```python
from build123d import *

# Parameters (mm, degrees)
F1_DEPTH = 12
F3_DEPTH = 90


with BuildPart() as f1:
    # F0 (on Front) → F1 (new body)
    with BuildSketch(Plane.XZ):
        Polygon((47.5, -67), (47.5, 0), (47.5, 67), (0, 67), (-47.5, 67), (-47.5, -67), align=None)
    extrude(amount=F1_DEPTH)

    # F2 (on face) → F3 (join)
    with BuildSketch(Plane.XZ.offset(12)):
        with BuildLine():
            Line((0, 5), (0, 0))
            Line((0, 0), (-4.8013158464, 0))
            ThreePointArc((-4.8013158464, 0), (-1.2386876382, -6.0708472044), (0, -13))
            ThreePointArc((0, -13), (12.7279220614, -7.7279220614), (18, 5))
            ThreePointArc((18, 5), (12.7279220614, 17.7279220614), (0, 23))
            Line((0, 23), (0, 5))
        make_face()
        with BuildLine():
            Line((-4.8013158464, 0), (0, 0))
            Line((0, 0), (0, 5))
            Line((0, 5), (0, 23))
            ThreePointArc((0, 23), (-5.397234005, 11.476680806), (-17.7049180328, 8.2459016393))
            ThreePointArc((-17.7049180328, 8.2459016393), (-17.8156486606, 7.5695647107), (-17.9005524862, 6.8895027624))
            ThreePointArc((-17.9005524862, 6.8895027624), (-10.6901851858, 4.7010550004), (-4.8013158464, 0))
        make_face()
        with BuildLine():
            ThreePointArc((0, -13), (-1.2386876382, -6.0708472044), (-4.8013158464, 0))
            Line((-4.8013158464, 0), (-7.550100402, 0))
            ThreePointArc((-7.550100402, 0), (-3.4675400893, -5.881167982), (-2.0003453113, -12.8885052096))
            ThreePointArc((-2.0003453113, -12.8885052096), (-1.0017250687, -12.9721046872), (0, -13))
        make_face()
        with BuildLine():
            Line((-7.550100402, 0), (-4.8013158464, 0))
            ThreePointArc((-4.8013158464, 0), (-10.6901851858, 4.7010550004), (-17.9005524862, 6.8895027624))
            ThreePointArc((-17.9005524862, 6.8895027624), (-17.9779647514, 5.8903838491), (-17.9996546887, 4.8885052096))
            ThreePointArc((-17.9996546887, 4.8885052096), (-12.3726305137, 3.3040864423), (-7.550100402, 0))
        make_face()
        with BuildLine():
            ThreePointArc((-2.0003453113, -12.8885052096), (-3.4675400893, -5.881167982), (-7.550100402, 0))
            Line((-7.550100402, 0), (-17.2916164658, 0))
            ThreePointArc((-17.2916164658, 0), (-11.6005749399, -8.76323585), (-2.0003453113, -12.8885052096))
        make_face()
        with BuildLine():
            Line((-17.2916164658, 0), (-7.550100402, 0))
            ThreePointArc((-7.550100402, 0), (-12.3726305137, 3.3040864423), (-17.9996546887, 4.8885052096))
            ThreePointArc((-17.9996546887, 4.8885052096), (-17.8141187186, 2.4198499502), (-17.2916164658, 0))
        make_face()
        with BuildLine():
            ThreePointArc((-17.7049180328, 8.2459016393), (-5.397234005, 11.476680806), (0, 23))
            ThreePointArc((0, 23), (-1.0017918512, 22.9721009647), (-2.0004782551, 22.888490343))
            ThreePointArc((-2.0004782551, 22.888490343), (-6.6776028044, 13.0131233652), (-17.2344944225, 10.1934768701))
            ThreePointArc((-17.2344944225, 10.1934768701), (-17.4968253692, 9.2262396998), (-17.7049180328, 8.2459016393))
        make_face()
        with BuildLine():
            ThreePointArc((-17.2344944225, 10.1934768701), (-6.6776028044, 13.0131233652), (-2.0004782551, 22.888490343))
            ThreePointArc((-2.0004782551, 22.888490343), (-11.523319194, 18.8279830328), (-17.2344944225, 10.1934768701))
        make_face()
    extrude(amount=F3_DEPTH)


solid = f1.part
```
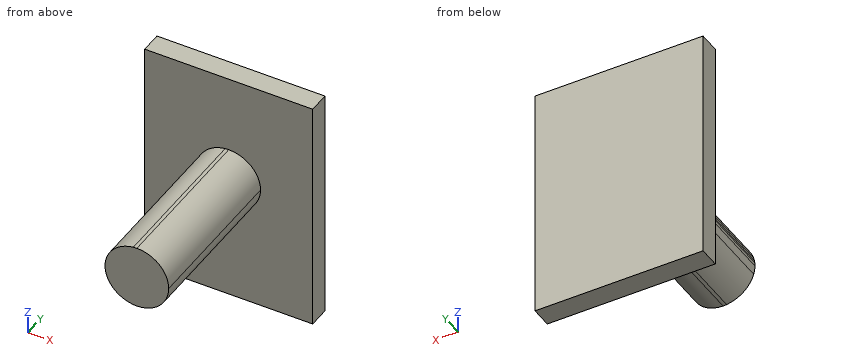
Design review of the part built by this model. Coordinates are the model's own, in mm. Coordinates: 2 decimals unless noted, no trailing zeros. Order: outer loops, then holes, each group sorted by start corner. A loop starts at its lowest first (then second) coordinate and runs counter-clockwise, first axis right, second up.
1) Wall thickness on line 1 along Y through (x, z) = (41, -47); line 2 along X through (y, z) = (-68.5, 18); line 3 along Z through (x, y) = (-11, -84): over which ranges is each line inside the solid? List them lowest first.
2) Take a section at B-B, the plane x = 13. Give the boundary of the cut face in (y, z), and give its area (3 significant figures).
3) Take a section at A-A, the plane y = -18. Give the boundary of the cut face in (x, z), and give its area (3 significant figures).
4) Take a section at D-D, the plane x = -26.5. Give the boundary of the cut face in (y, z).
5) Clearance check with flat-ended pins moving along their axes: pin 1 (10 mm diameter, centred on x = -33, z = 43, fed in from -Y); pin 2 (1 mm diameter, centred on x = -12, y = -43.5, fed in from -Z); pin 3 (12 mm diameter, centred on y = -44, z = 15, fed in from +X). State where each tip first meets the part, or that it passes through.
6) Take a section at C-C, the plane z = 14.5. Give the boundary of the cut face in (x, y), and give its area (3 significant figures).
Returned:
1. line 1: y = -12 to 0
1. line 2: x = -12.45 to 12.45
1. line 3: z = -9.25 to 19.25
2. outline: (-102, -7.45) - (-12, -7.45) - (-12, -67) - (0, -67) - (0, 67) - (-12, 67) - (-12, 17.45) - (-102, 17.45) - close
2. area: 3,850 mm2
3. outline: circle Ø36 at (0, 5)
3. area: 1,020 mm2
4. outline: (-12, -67) - (0, -67) - (0, 67) - (-12, 67) - close
5. pin 1: stops at y = -12
5. pin 2: stops at z = -8.85
5. pin 3: stops at x = 17.55
6. outline: (-47.5, -12) - (-15.29, -12) - (-15.29, -102) - (15.29, -102) - (15.29, -12) - (47.5, -12) - (47.5, 0) - (-47.5, 0) - close
6. area: 3,890 mm2
